Here's the drawing with two shaded views (mm, measured from the low corner). I have some questions. Give positions to 0.01 mm unless a question says otherwise; leave off trailing zeros. Loops run counter-clockwise (first coordinate to the right, second up) from the corner with the lowest first, then second, coordinate; pieces in that order, holes last. Notation, with made-up numbers: M 26,78.25 L 53,78.25 A20 cw 53,86.25 Z; hole C 28.25,13.5 d3. An arc over 180 degrees is marked long. Use CSV: the item, a comma, the result in double quotes.
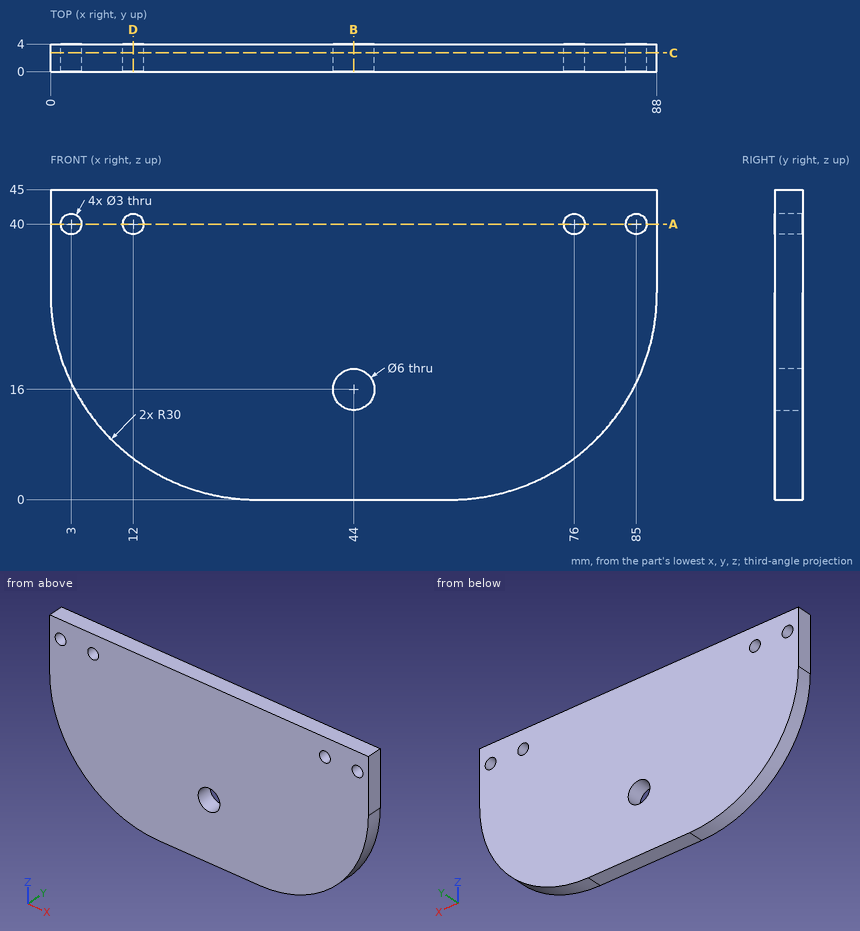
1. I want a section at B-B, the plane x = 44. List the corners of the cut face in (y, z) for me.
Outcome:
outline,"M 0,0 L 4,0 L 4,13 L 0,13 Z; M 0,19 L 4,19 L 4,45 L 0,45 Z"
2. I want a section at A-A, the plane z = 40. List the corners of the cut face in (x, y) for me.
Outcome:
outline,"M 0,0 L 1.5,0 L 1.5,4 L 0,4 Z; M 4.5,0 L 10.5,0 L 10.5,4 L 4.5,4 Z; M 13.5,0 L 74.5,0 L 74.5,4 L 13.5,4 Z; M 77.5,0 L 83.5,0 L 83.5,4 L 77.5,4 Z; M 86.5,0 L 88,0 L 88,4 L 86.5,4 Z"
3. I'm going to push flat-ended pins straight in: pin 1 Ø4 at (x, z) = (3, 40) entering from -Y; pin 2 Ø1 at (y, z) = (3.5, 11) entering from -X. Where does each tip first touch, or does it pass through?
Outcome:
pin 1,"y = 0"
pin 2,"x = 6.38"
4. I want a section at D-D, the plane x = 12. List the corners of the cut face in (y, z) for me.
Outcome:
outline,"M 0,6 L 4,6 L 4,38.5 L 0,38.5 Z; M 0,41.5 L 4,41.5 L 4,45 L 0,45 Z"
5. I want a section at C-C, the plane y = 2.7. List the corners of the cut face in (x, z) for me.
Outcome:
outline,"M 0,30 A30 ccw 30,0 L 58,0 A30 ccw 88,30 L 88,45 L 0,45 Z; hole C 3,40 d3; hole C 12,40 d3; hole C 44,16 d6; hole C 76,40 d3; hole C 85,40 d3"
6. Please list where these lines run through material, in increasing order: line 1 (X direction, y = 0.95, z = 40); line 2 (X direction, y = 2.55, z = 16); line 3 (Z direction, x = 75.5, y = 1.6).
Outcome:
line 1,"0 to 1.5, 4.5 to 10.5, 13.5 to 74.5, 77.5 to 83.5, 86.5 to 88"
line 2,"3.47 to 41, 47 to 84.53"
line 3,"5.63 to 38.59, 41.41 to 45"
